Build history of the part. All positions in model axes, mm. A direction names the side the tool comes from. Give positions to 0.01 mm unless a question says otherwise; leave off trailing zeros. Order: outer loops, then holes, each group sorted by start corner. A loop starts at its lowest first (then second) coordinate and runs counter-clockwise, first axis right, second up. Notation, with made-up numbers: (16.5, 55) - (43.5, 55) arc R5 ccw to (43.5, 63) - close; hole circle Ø7 at (-22.75, 76). An arc over 180 degrees is marked (long way). Write each question's results on one line, items separated by ' | '. Start each with the question number.
Autodesk Fusion 360 part; units mm, degrees
sketch "草图1" plane through (0, 0, 0) normal (0, 0, 1) x (1, 0, 0)
  line L0 (20, 20) -> (-20, 20)
  line L1 (-20, 20) -> (-20, -20)
  line L2 (-20, -20) -> (20, -20)
  line L3 (20, -20) -> (20, 20)
  line L4 (20, 20) -> (-20, -20) construction
  line L5 (-20, 20) -> (20, -20) construction
  dimension "d25" = 40
  dimension "d26" = 40
extrude "拉伸1" add sketch "草图1" along normal blind 6
fillet "圆角1" radius 4 4 edges at (-20, -20, 3) (20, -20, 3) (20, 20, 3) (-20, 20, 3)
sketch "草图2" plane through (0, 0, 6) normal (0, 0, 1) x (-1, 0, 0)
  arc A0 (16, -20) -> (20, -16) centre (16, -16) ccw
  line L0 (20, -16) -> (20, 16)
  arc A1 (20, 16) -> (16, 20) centre (16, 16) ccw
  line L1 (16, 20) -> (-16, 20)
  arc A2 (-16, 20) -> (-20, 16) centre (-16, 16) ccw
  line L2 (-20, 16) -> (-20, -16)
  arc A3 (-20, -16) -> (-16, -20) centre (-16, -16) ccw
  line L3 (-16, -20) -> (16, -20)
  point P0 (-10, -10)
  dimension "d31" = 10
  dimension "d32" = 10
hole "孔1" at (10, 10, 6) direction (0, 0, -1) diameter 3.4 depth 15 tip angle 118 counterbore diameter 6.5 counterbore depth 3.3
pattern_linear "R-阵列1" count 2 spacing 20 along (-1, 0, 0) count 2 spacing 20 along (0, -1, 0) of "孔1"
sketch "草图3" plane through (0, 0, 6) normal (0, 0, 1) x (-1, 0, 0)
  circle A0 centre (10, 10) radius 3.25
  circle A1 centre (-10, 10) radius 3.25
  circle A2 centre (10, -10) radius 3.25
  circle A3 centre (-10, -10) radius 3.25
  arc A4 (16, -20) -> (20, -16) centre (16, -16) ccw
  line L0 (20, -16) -> (20, 16)
  arc A5 (20, 16) -> (16, 20) centre (16, 16) ccw
  line L1 (16, 20) -> (-16, 20)
  arc A6 (-16, 20) -> (-20, 16) centre (-16, 16) ccw
  line L2 (-20, 16) -> (-20, -16)
  arc A7 (-20, -16) -> (-16, -20) centre (-16, -16) ccw
  line L3 (-16, -20) -> (16, -20)
  circle A8 centre (0, 0) radius 5.4
  dimension "d42" = 10.8
extrude "拉伸2" add sketch "草图3" along normal blind 1.8 contours A8
fillet "圆角2" radius 1 1 edges at (5.0346, -1.9527, 6)
sketch "草图4" plane through (0, 0, 7.8) normal (0, 0, 1) x (-1, 0, 0)
  circle A0 centre (0, 0) radius 5.4
  circle A1 centre (0, 0) radius 3.95
  dimension "d47" = 7.9
extrude "拉伸3" add sketch "草图4" along normal blind 18 contours A1
fillet "圆角3" radius 0.3 1 edges at (3.6827, -1.4284, 7.8)
chamfer "倒角1" distance 0.5 angle 45 1 edges at (3.6827, 1.4284, 25.8)
sketch "草图5" plane through (0, 0, 0) normal (0, 1, 0) x (1, 0, 0)
sketch "草图6" plane through (0, 0, 0) normal (0, 0, 1) x (1, 0, 0)
  line L0 (20, -3) -> (43, -3)
  line L1 (43, -3) -> (43, 3)
  line L2 (43, 3) -> (20, 3)
  line L3 (20, 3) -> (20, -3)
extrude "拉伸4" add sketch "草图6" along normal blind 6 and the other way blind 17
sketch "草图7" plane through (0, 3, 0) normal (0, 1, 0) x (-1, 0, 0)
  line L0 (-20, 0) -> (-20, 6)
  line L1 (-20, 6) -> (-43, 6)
  line L2 (-43, 6) -> (-43, -17)
  line L3 (-43, -17) -> (-20, -17)
  line L4 (-20, -17) -> (-20, 0)
  circle A0 centre (-31.5, -5.5) radius 5.25
  line L5 (0, 20) -> (0, 2.5)
  dimension "d57" = 10.5
  dimension "d58" = 31.5
  dimension "d59" = 11.5
extrude "拉伸5" cut sketch "草图7" against normal blind 6 contours A0
sketch "草图8" plane through (0, 3, 0) normal (0, 1, 0) x (-1, 0, 0)
  circle A0 centre (-31.5, -5.5) radius 5.25
  line L0 (-20, 0) -> (-20, 6)
  line L1 (-20, 6) -> (-43, 6)
  line L2 (-43, 6) -> (-43, -17)
  line L3 (-43, -17) -> (-20, -17)
  line L4 (-20, -17) -> (-20, 0)
  circle A1 centre (-31.5, 2.875) radius 1.7
  circle A2 centre (-31.5, -13.875) radius 1.7
  circle A3 centre (-39.875, -5.5) radius 1.7
  circle A4 centre (-23.125, -5.5) radius 1.7
  dimension "d62" = 3.4
  dimension "d64" = 3.125
  dimension "d67" = 11.5
  dimension "d68" = 3.4
  dimension "d69" = 3.125
  dimension "d70" = 11.5
  dimension "d71" = 3.4
  dimension "d72" = 3.4
  dimension "d73" = 3.125
  dimension "d74" = 3.125
  dimension "d75" = 11.5
  dimension "d76" = 11.5
extrude "拉伸7" cut sketch "草图8" against normal blind 6 contours A1 | A2 | A3 | A4
fillet "圆角4" radius 4 3 edges at (43, 0, 6) (43, 0, -17) (20, 0, -17)
equation "Base_Length = Base length"
equation "Base_Width = Base width"
equation "Base_Thickness = Base thickness"
equation "Base_Corner_Radius = Base corner radius"
equation "Hole_Pitch_X = M3 hole pitch X"
equation "Hole_Pitch_Y = M3 hole pitch Y"
equation "M3_Clearance_Diameter = M3 clearance hole diameter"
equation "Counterbore_Diameter = M3 socket-head counterbore diameter"
equation "Counterbore_Depth = M3 counterbore depth"
equation "Shaft_Diameter = Vertical printed shaft diameter"
equation "Shoulder_Diameter = Bearing inner-ring support shoulder diameter"
equation "Shoulder_Height = Bearing shoulder height"
equation "Shaft_Height = Shaft height above shoulder"
equation "Shoulder_Base_Fillet = Fillet between shoulder and base"
equation "Shaft_Shoulder_Fillet = Small fillet between shaft and shoulder"
equation "Shaft_Top_Chamfer = Shaft top lead-in chamfer"
equation "Bearing_Width = 608 bearing width"
equation "Bearing_Stack_Width = Two 608 bearings total width"
equation "Top_Retention_Hole_Diameter = Transverse retention hole diameter"
equation "Top_Retention_Hole_Height = Hole center height above shoulder"
equation "Axial_Clearance_Target = Target axial play under retention pin"
equation "Bearing_ID = 608 bearing nominal inner diameter"
equation "Bearing_OD = 608 bearing nominal outer diameter"
equation "Wheel_Base_Clearance_Target = Target wheel-to-base clearance"
equation "d25 = Base_Length"
equation "d26 = Base_Width"
equation "d27 = Base_Thickness"
equation "d30 = Base_Corner_Radius"
equation "d31 = ( Base_Length - Hole_Pitch_X ) / 2"
equation "d32 = ( Base_Width - Hole_Pitch_Y ) / 2"
equation "d34 = M3_Clearance_Diameter"
equation "d36 = Counterbore_Depth"
equation "d37 = Counterbore_Diameter"
equation "d40 = Hole_Pitch_X"
equation "d41 = Hole_Pitch_Y"
equation "d42 = Shoulder_Diameter"
equation "d43 = Shoulder_Height"
equation "d46 = Shoulder_Base_Fillet"
equation "d47 = Shaft_Diameter"
equation "d48 = Shaft_Height"
equation "d51 = Shaft_Shoulder_Fillet"
equation "d52 = Shaft_Top_Chamfer"
equation "d58 = ( 23 / 2 ) * 1 mm + 20 mm"
equation "d59 = ( 23 / 2 ) * 1 mm"
equation "d64 = ( ( 23 / 2 - 10.5 / 2 ) / 2 ) * 1 mm"
equation "d67 = ( 23 / 2 ) * 1 mm"
equation "d80 = Base_Corner_Radius"
Item 1: Cut at B-B, the plane x = 31.5. List the corners of the cut face in (y, z) (3 decimals).
Item 2: Two-plate mould, pull along X, no slides. Class faces 1 (the flat face through (-8.6, -11.4, 2.7)), 2 (the cylindrical face through (3.135, -2.404, 16.58)), 3 (the cylindrical face through (18.859, 18.797, 3.042)): +X half, -X half, draft (parallel to the pull), parting line (faces both ways), or undercut.
Item 3: Which spindle directions (+Z, -Z, +X, -X, +Y, -Y) get a long thin tool onto all of the face, cutting with end or side? Do faces 4 (the flat face through (20, -10, 3)), 5 (the flat face through (-20, 0, 3)), 6 (the flat face through (20, 9, 3)), 7 (the cylindrical face through (-10.143, -6.753, 4.327)). Say none if no direction does.
Item 4: Cut at D-D, the plane y = 0. List the corners of the cut face in (x, z) (3 decimals), then the cut area to 3 significant figures.
Item 5: Probe line 1 along X through (y, z) = (-10, 5.1); line 2 along Y through (x, z) = (10, 2.05). List the from-to ranges inside material, lowest first. Write a range as from..to.
Item 6: Cut at A-A, the plane x = -10. List the corners of the cut face in (y, z), then the cut area to 3 significant figures.
Item 7: Flat gauge pins, fed straight in: pin 1 Ø2 at (x, y) = (-10, -11) entering from +Z; pin 2 Ø12 at (y, z) = (-11, -2) entering from +X; pin 3 Ø5 at (x, y) = (9, 8.5) entering from +Z; pin 4 Ø4 at (x, z) = (17, -0.5) entering from +Y. Where does each tip first touch, or does it go through?
Values found:
1) outline: (-3, -17) - (3, -17) - (3, -15.575) - (-3, -15.575) - close; (-3, -12.175) - (3, -12.175) - (3, -10.75) - (-3, -10.75) - close; (-3, -0.25) - (3, -0.25) - (3, 1.175) - (-3, 1.175) - close; (-3, 4.575) - (3, 4.575) - (3, 6) - (-3, 6) - close
2) face 1: undercut | face 2: parting line | face 3: +X half
3) face 4: +Z, -Z, +X, -Y | face 5: +Z, -Z, -X, +Y, -Y | face 6: +Z, -Z, +X, +Y | face 7: +Z
4) outline: (-20, 0) - (20, 0) - (20, -13) arc R4 ccw to (24, -17) - (39, -17) arc R4 ccw to (43, -13) - (43, 2) arc R4 ccw to (39, 6) - (6.4, 6) arc R1 cw to (5.4, 7) - (5.4, 7.8) - (4.25, 7.8) arc R0.3 cw to (3.95, 8.1) - (3.95, 25.3) - (3.45, 25.8) - (-3.45, 25.8) - (-3.95, 25.3) - (-3.95, 8.1) arc R0.3 cw to (-4.25, 7.8) - (-5.4, 7.8) - (-5.4, 7) arc R1 cw to (-6.4, 6) - (-20, 6) - close; hole circle Ø3.4 at (23.125, -5.5); hole circle Ø10.5 at (31.5, -5.5); hole circle Ø3.4 at (31.5, -13.875); hole circle Ø3.4 at (31.5, 2.875); hole circle Ø3.4 at (39.875, -5.5) | area: 798 mm2
5) line 1: x = -20..-13.25, -6.75..6.75, 13.25..20 | line 2: y = -20..-11.7, -8.3..8.3, 11.7..20
6) outline: (-20, 0) - (-11.7, 0) - (-11.7, 2.7) - (-13.25, 2.7) - (-13.25, 6) - (-20, 6) - close; (-8.3, 0) - (8.3, 0) - (8.3, 2.7) - (6.75, 2.7) - (6.75, 6) - (-6.75, 6) - (-6.75, 2.7) - (-8.3, 2.7) - close; (11.7, 0) - (20, 0) - (20, 6) - (13.25, 6) - (13.25, 2.7) - (11.7, 2.7) - close | area: 179 mm2
7) pin 1: stops at z = 2.7 | pin 2: stops at x = 20 | pin 3: stops at z = 6 | pin 4: stops at y = 20
